Geometry: final body of the model. Coordinates: model frame, mm. Give positions to 0.01 mm unless a question says otherwise; leave off trailing zeros. Write each loop counter-clockwise with the first axis right and the second up, starting at its lowest first coordinate (ties: lowest second). Pieces come first, ordered by that corner, then holes. Notation, with made-up numbers: (61.25, 46) -> (100.25, 46) arc R12 cw to (100.25, 51) -> close; hole circle Ø10 at (31.25, 10). An arc over 180 degrees is marked (long way). Answer in a Markdown table with one row per item. Add a question column.
from build123d import *

# Parameters (mm, degrees)
REVOLVE6_ANGLE          = 180.0000000000004
CUT_EXTRUDE1_DEPTH      = 581.8775086022882
CUT_EXTRUDE1_DEPTH_BACK = 581.8775086022882
SKETCH2_R               = 5.5562499999999995


with BuildPart() as part:
    # Sketch1 → Revolve6 (revolve)
    with BuildSketch(Plane.XY):
        with BuildLine():
            Line((-228.59999999999997, 0), (-226.69500000000002, 0))
            ThreePointArc((-226.69500000000002, 0), (1.388e-14, 226.69500000000002), (226.69500000000002, 0))
            Line((226.69500000000002, 0), (228.59999999999997, 0))
            ThreePointArc((228.59999999999997, 0), (1.4e-14, 228.59999999999997), (-228.59999999999997, 0))
        make_face()
    revolve(axis=Axis((0, 0, 0), (1, 0, 0)), revolution_arc=REVOLVE6_ANGLE)

    # Sketch2 → Cut-Extrude1 (cut, two sides: drawn at the far end of the back side and taken through both)
    with BuildSketch(Plane(origin=(5.98e-15, 3.56628e-12, -253.99999999999983), x_dir=(-0.9340477296722021, -0.3571482027033107, -2.4939525698799316e-15), z_dir=(0, -6.98e-15, 1)).offset(-CUT_EXTRUDE1_DEPTH_BACK)):
        with Locations(Location((6.4581e-13, 1.67225e-12, 0), (0, 0, 249.074839669))):
            Circle(SKETCH2_R)
    extrude(amount=CUT_EXTRUDE1_DEPTH + CUT_EXTRUDE1_DEPTH_BACK, mode=Mode.SUBTRACT)

    # Mirror1: part across plane


with BuildPart() as part_1:
    add(part.part)
    add(part.part.mirror(Plane.XY))


solid = part_1.part
Q1. Contact query for flat-ended pins moving along their axis: pin 1 Ø4 at (y, z) = (-4.5, 10.5) entering from +X; pin 2 Ø5 at (x, z) = (146.5, -128) entering from +Y; pin 3 Ø4 at (y, z) = (-80.5, 43.5) entering from +X. Output: stop coordinate, or through.
Q2. Line query: probe 1 along X at (y, z) = (145, 17); probe 2 along Z at (x, y) = (77, -113); probe 3 along Z at (x, y) = (102, 142.5). Output: solid intervals per line, ascending. Write a range as from..to.
Q3. Section A-A on x = -45. Return loops of the section in (y, z).
Q4. Section B-B on z = 101. Return loops of the section in (x, y), and give its area (3 significant figures).
Checks:
| question | item | result |
|---|---|---|
| 1 | pin 1 | x = 228.41 |
| 1 | pin 2 | y = 124.01 |
| 1 | pin 3 | x = 210.35 |
| 2 | probe 1 | -175.91..-173.43, 173.43..175.91 |
| 2 | probe 2 | -183.19..-180.81, 180.81..183.19 |
| 2 | probe 3 | -146.79..-143.81, 143.81..146.79 |
| 3 | outline | circle Ø448.25 at (0, 0); hole circle Ø444.37 at (0, 0) |
| 4 | outline | circle Ø410.16 at (0, 0); hole circle Ø405.9 at (0, 0) |
| 4 | area | 2,720 mm^2 |
